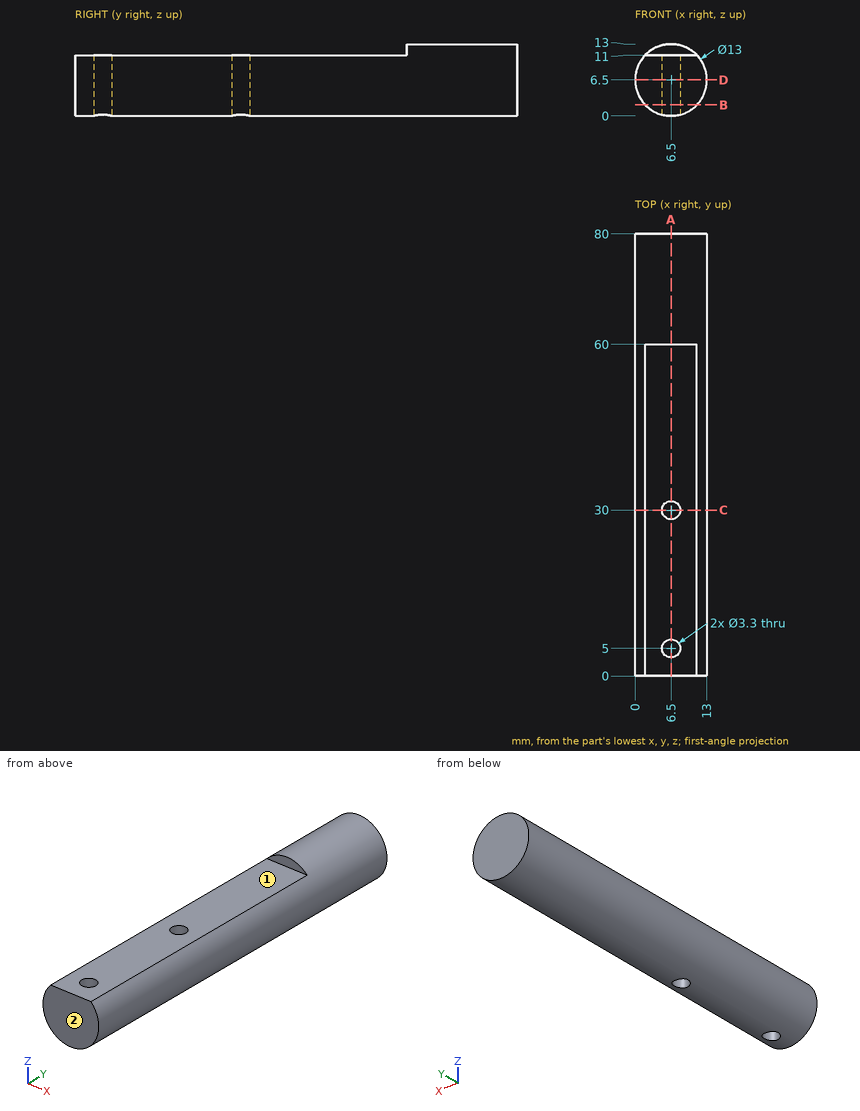
Can you work these out from the drawing? Everything is in mm from the part's minimum corner. A direction names the side the tool comes from. Round coordinates to 2 decimals unless told otherwise and drop trailing zeros. Loops run counter-clockwise (first coordinate to the right, second up) from the corner with the lowest first, then second, coordinate; pieces in that order, holes last. Notation, with made-up numbers: (83, 37) -> (89, 37) arc R14 ccw to (89, 50) -> close; hole circle Ø6 at (62, 5). An arc over 180 degrees is marked (long way). One line per question, with ' | ' between items.
(1) If we section it at B-B on z = 2: List the corners of the cut face in (x, y) for me.
Model answer:
outline: (1.81, 0) -> (11.19, 0) -> (11.19, 80) -> (1.81, 80) -> close; hole circle Ø3.3 at (6.5, 5); hole circle Ø3.3 at (6.5, 30)
(2) If I drill on probe 1 along Y at (x, z) = (6.5, 5.5); probe 2 along Y at (x, z) = (5.25, 2); probe 3 along X at (y, z) = (42, 2), over which ranges is the centre line in solid material (lowest first)?
Model answer:
probe 1: y = 0 to 3.35, 6.65 to 28.35, 31.65 to 80 | probe 2: y = 0 to 3.92, 6.08 to 28.92, 31.08 to 80 | probe 3: x = 1.81 to 11.19
(3) If we section it at D-D on z = 6.5: List the corners of the cut face in (x, y) for me, and give its area (3 significant figures).
Model answer:
outline: (0, 0) -> (13, 0) -> (13, 80) -> (0, 80) -> close; hole circle Ø3.3 at (6.5, 5); hole circle Ø3.3 at (6.5, 30) | area: 1,020 mm^2
(4) If we section it at A-A on x = 6.5: List the corners of the cut face in (y, z) for me.
Model answer:
outline: (0, 0) -> (3.35, 0) -> (3.35, 11) -> (0, 11) -> close; (6.65, 0) -> (28.35, 0) -> (28.35, 11) -> (6.65, 11) -> close; (31.65, 0) -> (80, 0) -> (80, 13) -> (60, 13) -> (60, 11) -> (31.65, 11) -> close
(5) For the marked faces 1 and 2, which set-ups out of +Z, -Z, +X, -X, +Y, -Y let a thin tool reach every point of the face, with its end or its side?
Model answer:
face 1: +Z, +X, -X, -Y | face 2: +Z, -Z, +X, -X, -Y
(6) For pin 1 Ø7.5 at (x, y) = (8, 20) entering from +Z; pin 2 Ø1 at (x, y) = (7.5, 62) entering from +Z; pin 3 Ø1.6 at (x, z) = (4.5, 12) entering from -Y, each with a flat end and sliding along its axis, tell me the tip position at first contact or that it passes through.
Model answer:
pin 1: stops at z = 11 | pin 2: stops at z = 12.98 | pin 3: stops at y = 60
(7) If we section it at C-C on y = 30: List the corners of the cut face in (x, z) for me, and give its area (3 significant figures).
Model answer:
outline: (1.81, 11) arc R6.5 ccw to (4.85, 0.21) -> (4.85, 11) -> close; (8.15, 0.21) arc R6.5 ccw to (11.19, 11) -> (8.15, 11) -> close | area: 83.7 mm^2
